Can you work these out from the model? Positions are in its coordinate system, mm. Face numbers are marked on the shaded views. A direction names the side the tool comes from. Round coordinates to 2 decimals unless told otherwise and drop trailing zeros. Order: outer loops, then holes, each group sorted by start corner. A loop starts at its lowest first (then second) coordinate and runs counter-clockwise, first axis right, second up. Notation, with made-up numbers: (50, -1) -> (95, -1) arc R18 ccw to (95, 25) -> close; hole circle Ø5 at (61, 70). An arc over 180 degrees is marked (long way). Use a Markdown table: item, result. Add a question column.
Q1. If we section it at A-A on y = 0: List the corners of the cut face in (x, z) for me, plus the area to 3 significant figures.
Q2. For the marked faces 1, 2 and 3, which set-ups out of +Z, -Z, +X, -X, +Y, -Y let a thin tool reach every point of the face, with its end or its side?
Q3. I need wall thicknesses on line 1 along X through (y, z) = (-0.75, -3); line 2 along Y through (x, z) = (4, 1.5); line 3 along Y through (x, z) = (22.25, 1.75). Which ranges of each line are inside material? Lowest first, please. Write a range as [from, to].
Q4. If we section it at D-D on y = -3: List the corners of the cut face in (x, z) for me.
Q5. I'm going to push flat-ended pins straight in: pin 1 Ø2 at (y, z) = (-2, -2.5) entering from +X; pin 2 Ø3 at (x, y) = (20, 3) entering from +Z. Where does each tip first touch, or does it pass through?
Q6. If we section it at C-C on x = 15.75: List the corners of the cut face in (y, z) for me.
Autodesk Inventor part; units mm, degrees
ref_plane "Startebene" through (0, 0, 0) normal (1, 0, 0) x (0, 1, 0)
ref_plane "XZ Plane" through (0, 0, 0) normal (0, 1, 0) x (-1, 0, 0)
ref_plane "XY Plane" through (0, 0, 0) normal (0, 0, 1) x (1, 0, 0)
sketch "Hauptskizze" plane through (0, 0, 0) normal (0, 0, 1) x (1, 0, 0)
  line L0 (0, 0) -> (25, 0)
  line L1 (0, 0) -> (0, 2.5)
  line L2 (0, 2.5) -> (5, 2.5)
  line L3 (5, 3.75) -> (20, 3.75)
  line L4 (25, 2.5) -> (25, 0)
  line L5 (20, 2.5) -> (25, 2.5)
  line L6 (5, 2.5) -> (5, 3.75)
  line L7 (20, 3.75) -> (20, 2.5)
  dimension "d3" = 5
  dimension "d5" = 7.5
  dimension "d14" = 5
revolve "Umdrehung1" add sketch "Hauptskizze" angle 360 about axis through (0, 0, 0) along (1, 0, 0)
chamfer "Fase3" distance 0.5 angle 45 1 edges at (25, -2.5, 0) measured on face at (21.6667, 2.4676, -0.401)
chamfer "Fase1" distance 0.5 angle 45 1 edges at (0, -2.5, 0) measured on face at (1.6667, 2.4676, -0.401)
properties part number "Welle 5x4+7.5x15+5x4" material "Messing, weicher Gelbton"
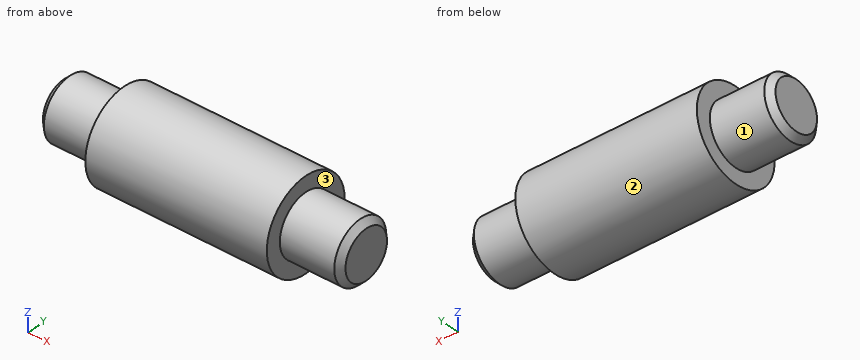
Answer below:
| question | item | result |
|---|---|---|
| 1 | outline | (0, -2) -> (0.5, -2.5) -> (5, -2.5) -> (5, -3.75) -> (20, -3.75) -> (20, -2.5) -> (24.5, -2.5) -> (25, -2) -> (25, 2) -> (24.5, 2.5) -> (20, 2.5) -> (20, 3.75) -> (5, 3.75) -> (5, 2.5) -> (0.5, 2.5) -> (0, 2) -> close |
| 1 | area | 162 mm² |
| 2 | face 1 | -X |
| 2 | face 2 | +X, -X |
| 2 | face 3 | +X |
| 3 | line 1 | [5, 20] |
| 3 | line 2 | [-2, 2] |
| 3 | line 3 | [-1.79, 1.79] |
| 4 | outline | (5, -2.25) -> (20, -2.25) -> (20, 2.25) -> (5, 2.25) -> close |
| 5 | pin 1 | x = 24.8 |
| 5 | pin 2 | z = 3.44 |
| 6 | outline | circle Ø7.5 at (0, 0) |
